Could you check a few things on this drawing? It's one solid part, dimensions in mm from its lowest x, y, z. Coordinates: 2 decimals unless noted, no trailing zeros. Write each loop counter-clockwise with the first axis right and the second up, starting at its lowest first coordinate (ties: lowest second). Pieces come first, ordered by that corner, then holes. Notation, with made-up numbers: M -4,86.25 L 30,86.25 A16 ccw 30,107.25 Z; hole C -18,5 d8. An arc over 180 degrees is marked long. Use a Markdown table: item, result.
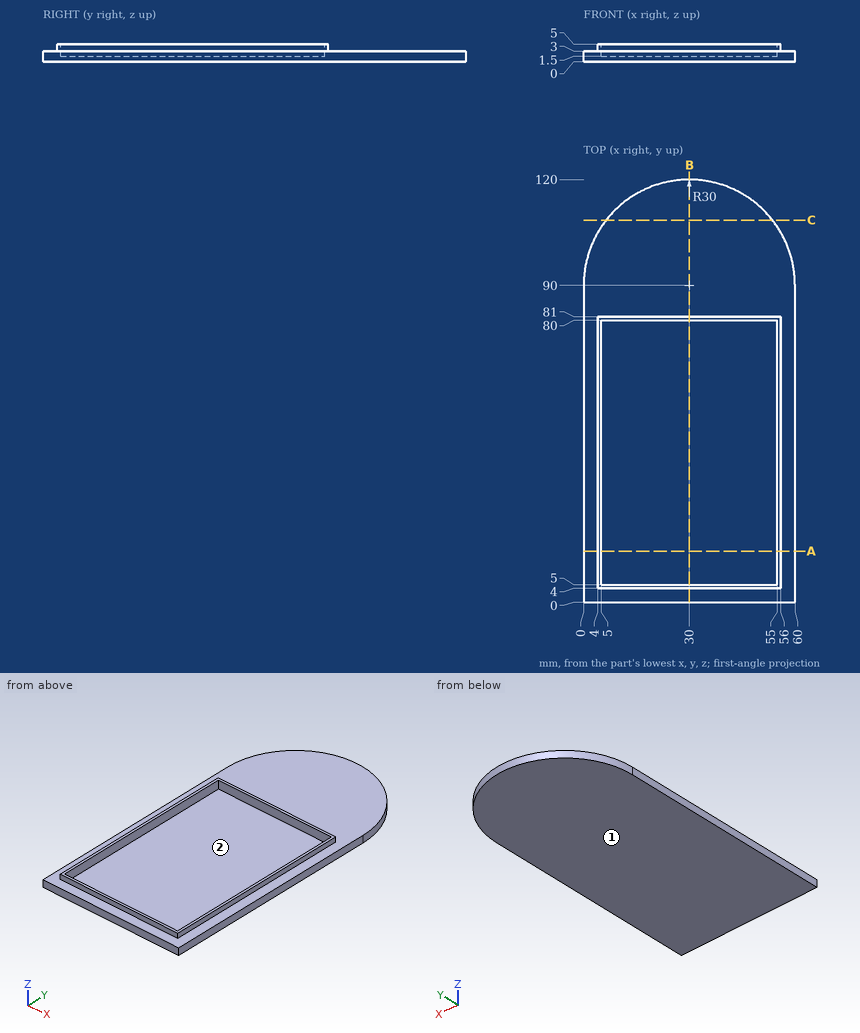
1. I need wall thicknesses on probe 1 along X at (y, z) = (54.5, 1.95); probe 2 along X at (y, z) = (55.5, 3.85); probe 3 along Y at (x, z) = (6, 4.6). Which ranges of each line are inside material? Lowest first, please.
Answers follow:
| item | result |
|---|---|
| probe 1 | x = 0 to 5, 55 to 60 |
| probe 2 | x = 4 to 5, 55 to 56 |
| probe 3 | y = 4 to 5, 80 to 81 |
2. Suppose I cut it at A-A on y = 14.5. Write out the boundary of the cut face in (x, z), and give its area (3 significant figures).
Answers follow:
| item | result |
|---|---|
| outline | M 0,0 L 60,0 L 60,3 L 56,3 L 56,5 L 55,5 L 55,1.5 L 5,1.5 L 5,5 L 4,5 L 4,3 L 0,3 Z |
| area | 109 mm2 |
3. Suppose I cut it at C-C on y = 108.5. Write out the boundary of the cut face in (x, z), and give its area (3 significant figures).
Answers follow:
| item | result |
|---|---|
| outline | M 6.38,0 L 53.62,0 L 53.62,3 L 6.38,3 Z |
| area | 142 mm2 |
4. Will these pins go through, and if not, where does the flat tip stop? pin 1 Ø1.5 at (y, z) = (14.5, 1.5) entering from -X; pin 2 Ø1.6 at (x, z) = (22.5, 4.5) entering from -Y; pin 3 Ø15 at (x, y) = (21.5, 34.5) entering from +Z; pin 4 Ø1.6 at (y, z) = (45, 4.5) entering from +X.
Answers follow:
| item | result |
|---|---|
| pin 1 | stops at x = 0 |
| pin 2 | stops at y = 4 |
| pin 3 | stops at z = 1.5 |
| pin 4 | stops at x = 56 |
5. We'd pull the mould along Y, two halves only. Please class the marked faces 1 and 2: +Y half, -Y half, draft (parallel to the pull), parting line (faces both ways), or undercut.
Answers follow:
| item | result |
|---|---|
| face 1 | draft |
| face 2 | undercut |
6. Suppose I cut it at B-B on x = 30. Write out the boundary of the cut face in (y, z).
Answers follow:
| item | result |
|---|---|
| outline | M 0,0 L 120,0 L 120,3 L 81,3 L 81,5 L 80,5 L 80,1.5 L 5,1.5 L 5,5 L 4,5 L 4,3 L 0,3 Z |
